The model under review builds one solid part; all positions refer to its coordinate system, in mm. A direction names the side the tool comes from. Give positions to 0.01 mm unless a question says otherwise; leave off trailing zeros. Write each loop counter-clockwise with the first axis right and the second up, starting at its lowest first coordinate (ties: lowest second). Pieces come first, ordered by that corner, then holes.
Autodesk Inventor part; units mm, degrees
ref_plane "YZ Plane" through (0, 0, 0) normal (1, 0, 0) x (0, 1, 0)
ref_plane "XZ Plane" through (0, 0, 0) normal (0, 1, 0) x (-1, 0, 0)
ref_plane "XY Plane" through (0, 0, 0) normal (0, 0, 1) x (1, 0, 0)
sketch "草图1" plane through (0, 0, 0) normal (1, 0, 0) x (0, 1, 0)
  line L0 (600, 25) -> (-600, 25)
  line L1 (-600, 25) -> (-600, -25)
  line L2 (-600, -25) -> (600, -25)
  line L3 (600, -25) -> (600, 25)
  line L4 (600, 25) -> (-600, -25) construction
  line L5 (-600, 25) -> (600, -25) construction
  point P0 (0, 0)
  dimension "d0" = 1200
  dimension "d1" = 50
extrude "拉伸1" add sketch "草图1" along normal mid plane 15
sketch "草图2" plane through (7.5, 0, 0) normal (1, 0, 0) x (0, 0, -1)
  line L0 (-25, 600) -> (-25, -600)
  line L1 (25, -600) -> (25, 600)
  line L2 (-25, 600) -> (25, 600)
  line L3 (25, 600) -> (25, 550)
  line L4 (25, 550) -> (-25, 550)
  line L5 (-25, 550) -> (-25, 600)
  line L6 (-25, -600) -> (25, -600)
  line L7 (25, -600) -> (25, -550)
  line L8 (25, -550) -> (-25, -550)
  line L9 (-25, -550) -> (-25, -600)
  point P0 (0, 0)
  point P1 (-25, -550)
  point P2 (-25, 550)
extrude "拉伸2" add sketch "草图2" along normal blind 50 contours L2 L1 L4 L0 | L8 L1 L6 L0
sketch "草图3" plane through (-7.5, 0, 0) normal (-1, 0, 0) x (0, 0, 1)
  line L0 (-25, 600) -> (-25, -600)
  line L1 (-25, -600) -> (-5, -600)
  line L2 (-25, -600) -> (25, -600)
  line L3 (25, -600) -> (5, -600)
  line L4 (-5, -600) -> (-5, 600)
  line L5 (25, 600) -> (-25, 600)
  line L6 (5, 400) -> (5, -600)
  line L7 (25, 550) -> (25, -550)
  line L8 (5, 400) -> (5, 600)
  line L9 (-25, 600) -> (25, 600)
  point P0 (0, 0)
  point P1 (5, 500)
extrude "拉伸3" cut sketch "草图3" against normal blind 5 contours L5 L8 L6 L2 L4
properties part number "竖直滑台"
1) The part is to be moulded in two halves that separate along Y. For faces 1 (the flat face through (7.5, -8, 0)), 2 (the flat face through (25, -600, 0)), 3 (the flat face through (-7.5, -8, 15)), say which applies: +Y half, -Y half, draft (parallel to the pull), parting line (faces both ways), or undercut.
2) Insertion check: pin 1 (11 mm diameter, centred on y = -75, z = 0.5, fed in from -X); pin 2 (15 mm diameter, centred on y = 83, z = -6.5, fed in from +X). Each pin has a flat end and moves straight along its axis. Give the tip position at first contact, or say it passes through.
3) Consider section C-C, the plane y = -188. Give the boundary of the cut face in (x, z), then the cut area to 3 significant figures.
4) Tool access review of faces 4 (the flat face through (32, 550, 0)), 5 (the flat face through (3, -3, -25)): name each direction out of +Z, -Z, +X, -X, +Y, -Y from which nothing blocks a thin tool from reaching the whole face with its end or side.
5) Consider section A-A, the plane x = 34. Give the boundary of the cut face in (y, z).
6) To check wall thickness, follow probe 1 along Y at (x, z) = (48, 12); probe 2 along X at (y, z) = (-98, 11); probe 3 along X at (y, z) = (272, 0). State the ranges of each line that lie inside material, in increasing order.
7) Consider section B-B, the plane z = -13. Give the boundary of the cut face in (x, y).
Answer block:
1. face 1: undercut
1. face 2: -Y half
1. face 3: draft
2. pin 1: stops at x = -7.5
2. pin 2: stops at x = 7.5
3. outline: (-7.5, -25) - (7.5, -25) - (7.5, 25) - (-7.5, 25) - (-7.5, 5) - (-2.5, 5) - (-2.5, -5) - (-7.5, -5) - close
3. area: 700 mm2
4. face 4: +Z, -Z, +X
4. face 5: -Z, +X, -X, +Y, -Y
5. outline: (-600, -25) - (-550, -25) - (-550, 25) - (-600, 25) - close; (550, -25) - (600, -25) - (600, 25) - (550, 25) - close
6. probe 1: y = -600 to -550, 550 to 600
6. probe 2: x = -7.5 to 7.5
6. probe 3: x = -2.5 to 7.5
7. outline: (-7.5, -600) - (57.5, -600) - (57.5, -550) - (7.5, -550) - (7.5, 550) - (57.5, 550) - (57.5, 600) - (-7.5, 600) - close
